Geometry: final body of the model. Coordinates: model frame, mm. A direction names the side the tool comes from. Round coordinates to 2 decimals unless told otherwise and drop trailing zeros. Loops run counter-clockwise (first coordinate to the right, second up) from the corner with the lowest first, then second, coordinate; pieces in that order, holes last. Notation, with made-up numbers: (-19, -17) - (28, -17) arc R26 cw to (28, 22) - close; hole circle Ø1 at (50.25, 18.5). An arc over 180 degrees is marked (long way). Write item = value, one per line. Start each with the question number.
Item 1: Draft query along Z for faces 1 (the flat face through (-44.45, 0, 75)), 2 (the flat face through (-30, 20, 152.4)), 3 (the flat face through (-1, 1, 0)). Return one class per face: pulls with the +Z half, pulls with the -Z half, needs draft (parallel to the pull), parting line crosses it, or undercut.
Item 2: Section D-D (z = 13.5). Return loops of the section in (x, y).
Item 3: First-contact query: pin 1 (4 mm diameter, centred on x = -33.5, y = 30.5, fed in from -Z); pin 2 (4 mm diameter, centred on x = -4, y = -31.5, fed in from +Z). Flat tips, straight axial feed; report the tip coordinate or a pass-through.
Item 4: Section B-B (x = 0). Return loops of the section in (y, z) (3 decimals), plus the area to 3 significant figures.
Item 5: Line query: line 1 (X direction, y = 0, z = 130) (3 decimals); line 2 (Z direction, x = 15, y = 16.5). Output: solid intervals per line, ascending. Write a range as from..to.
Item 6: Access query for faces 4 (the cylindrical face through (11.59, -15.12, 152.93)), 5 (the flat face through (0, 44.45, 75)). Directions: +Z, -Z, +X, -X, +Y, -Y. A direction counts if a zero-diameter tool reaches every point of the face in a straight line with its end or side. Return the directions, or none.
Item 7: Section A-A (z = 139). Return loops of the section in (x, y) (3 decimals).
Solid Edge part; units mm, degrees
sketch "Sketch1" plane through (0, 0, 0) normal (0, 0, 1) x (1, 0, 0)
  line L0 (-44.45, -44.45) -> (44.45, -44.45)
  line L1 (44.45, -44.45) -> (44.45, 44.45)
  line L2 (44.45, 44.45) -> (-44.45, 44.45)
  line L3 (-44.45, 44.45) -> (-44.45, -44.45)
extrude "Protrusion1" add sketch "Sketch1" along normal blind 152.4
fillet "Round_1" radius 12.7 4 edges at (44.45, -44.45, 76.2) (-44.45, -44.45, 76.2) (44.45, 44.45, 76.2) (-44.45, 44.45, 76.2)
sketch "Sketch2" plane through (0, 0, 152.4) normal (0, 0, 1) x (0, 1, 0)
  circle A0 centre (0, 0) radius 34.925
extrude "ExtrudedCutout_1" cut sketch "Sketch2" against normal blind 38.1
sketch "Sketch3" plane through (0, 0, 152.4) normal (0, 0, 1) x (0, 1, 0)
  circle A0 centre (0, 0) radius 19.05
extrude "Protrusion2" add sketch "Sketch3" against normal up to next
sketch "Sketch4" plane through (0, 0, 152.4) normal (0, 0, 1) x (0, 1, 0)
  circle A0 centre (0, 0) radius 19.05
extrude "ExtrudedProtrusion_3" add sketch "Sketch4" along normal blind 38.1
Taken from the geometry:
q1.face_1 = needs draft
q1.face_2 = pulls with the +Z half
q1.face_3 = pulls with the -Z half
q2.outline = (-44.45, -31.75) arc R12.7 ccw to (-31.75, -44.45) - (31.75, -44.45) arc R12.7 ccw to (44.45, -31.75) - (44.45, 31.75) arc R12.7 ccw to (31.75, 44.45) - (-31.75, 44.45) arc R12.7 ccw to (-44.45, 31.75) - close
q3.pin_1 = 0
q3.pin_2 = 114.3
q4.outline = (-44.45, 0) - (44.45, 0) - (44.45, 152.4) - (34.925, 152.4) - (34.925, 114.3) - (19.05, 114.3) - (19.05, 190.5) - (-19.05, 190.5) - (-19.05, 114.3) - (-34.925, 114.3) - (-34.925, 152.4) - (-44.45, 152.4) - close
q4.area = 13,800 mm^2
q5.line_1 = -44.45..-34.925, -19.05..19.05, 34.925..44.45
q5.line_2 = 0..114.3
q6.face_4 = +Z
q6.face_5 = +Z, -Z, +X, -X, +Y
q7.outline = (-44.45, -31.75) arc R12.7 ccw to (-31.75, -44.45) - (31.75, -44.45) arc R12.7 ccw to (44.45, -31.75) - (44.45, 31.75) arc R12.7 ccw to (31.75, 44.45) - (-31.75, 44.45) arc R12.7 ccw to (-44.45, 31.75) - close; circle Ø38.1 at (0, 0); hole circle Ø69.85 at (0, 0)
